Here's how the part is built. I have some questions about the finished solid (model axes, mm). A direction names the side the tool comes from. Round coordinates to 2 decimals unless told otherwise and drop trailing zeros. Write each loop counter-clockwise with the first axis right and the second up, starting at its lowest first coordinate (ties: lowest second). Pieces come first, ordered by that corner, then holes. Notation, with made-up numbers: (23, -0.75) -> (65, -0.75) arc R22 cw to (65, 29.25) -> close; hole circle Ø10 at (55, -7.75). An arc over 180 degrees is marked (long way). Answer in a Markdown table with one row per item. Add a question column.
from build123d import *

# Parameters (mm, degrees)
F4_R     = 3.4
F5_DEPTH = 75.0134427933
F6_SIZE  = 1.5
F7_COUNT = 3


with BuildPart() as f1:
    # F0 (on Front) → F1 (revolve)
    with BuildSketch(Plane.XZ):
        Polygon((-9.15, 1), (-9.15, 25), (-14, 25), (-25, 14.5), (-25, 10.5), (-14, 0), (-10.15, 0), (-10.15, 1), align=None)
    revolve(axis=Axis((0, 0, 12.5), (0, 0, -1)))

    # F2 (on Front) → F3 (revolve)
    with BuildSketch(Plane.XZ):
        Polygon((-35.584796918, -20.8697111031), (-14.8705245175, 0.8309552212), (-10.4189875067, 5.4944701849), (-15.0484629892, 9.9135149637), (-19.5, 5.25), (-40.2142724005, -16.4506663243), align=None)
    revolve(axis=Axis((-29.8571362002, 0, -5.6003331622), (0.6904757467, 0, 0.7233555441)))

    # F4 (on face) → F5 (cut, through all)
    with BuildSketch(Plane(origin=(-27.3888669951, 0, -28.6930987567), x_dir=(0.7233555441, 0, -0.6904757467), z_dir=(-0.6904757467, 0, -0.7233555441))):
        with Locations((-17.7304307809, 0)):
            Circle(F4_R)
    extrude(amount=-F5_DEPTH, mode=Mode.SUBTRACT)

    # F6
    f6_edges = [f1.edges().sort_by_distance(p)[0] for p in [
        (-44.843748, 0, -12.031622),
    ]]
    chamfer(f6_edges, length=F6_SIZE)

    # F7: F1 ×3 about axis
    f7_axis = Axis((0, 0, 14.5), (0, 0, -1))


with BuildPart() as f1_1:
    add(f1.part)
    for i in range(1, F7_COUNT):
        add(f1.part.rotate(f7_axis, i * 360 / F7_COUNT))


solid = f1_1.part
Item 1: If we mould it in two halves opening along X, with no side actions, what happens to faces 3 (the conical face through (-14.01, 4.412, 24.343)), 4 (the cylindrical face through (12.7, -24.61, -7.85)), 5 (the flat face through (9.399, 4.213, 0))? For each: pulls with the +X half, pulls with the -X half, needs draft (parallel to the pull), parting line crosses it, or undercut.
Item 2: If we section it at C-C on z = 18: Please give me the cut outline in (x, y), then the cut area to 3 significant figures.
Item 3: I need wall thicknesses on line 1 along Y through (x, z) = (-35.5, -11.5); line 2 along Y through (x, z) = (0, 14); line 3 along Y through (x, z) = (19, -14). Which ranges of each line are inside material? Lowest first, please. Write a range as from..to.
Item 4: For P1, Ø8, axis at y = -5.5, z = -1, coming from the -X side; P2, Ø3, axis at x = -32.5, z = 2, coming from the +Y side; P3, Ø3, axis at y = 9, z = 13.5, coming from the +X side, each with a flat end and sliding along its axis, tell me the tip position at first contact or that it passes through.
Item 5: On a 3-axis mill with a long thin cutter (end or side, diameter ignored), from which of +Z, -Z, +X, -X, +Y, -Y can I reach the whole of each face in a straight line? I mean faces 1 (the flat face through (3, -9, 25)), 2 (the conical face through (9.691, 16.882, 5.217)). Say none if no direction works.
Item 6: If we section it at A-A on x = 0: Please give me the cut outline in (y, z).
Item 7: If we section it at D-D on z = -8.5: Give the number of separate pieces and of enclosed holes in the cut face, then the cut area to 3 significant figures.
Item 8: If we section it at B-B on y = 0: Please give me the cut outline in (x, z).
Results list:
| question | item | result |
|---|---|---|
| 1 | face 3 | parting line crosses it |
| 1 | face 4 | undercut |
| 1 | face 5 | needs draft |
| 2 | outline | circle Ø42.67 at (0, 0); hole circle Ø18.3 at (0, 0) |
| 2 | area | 1,170 mm² |
| 3 | line 1 | -6.4..-3.4, 3.4..6.4 |
| 3 | line 2 | -25..-9.15, 9.15..25 |
| 3 | line 3 | -38.43..-37.06, -28.58..-24.84, 24.84..28.58, 37.06..38.43 |
| 4 | P1 | x = -36.26 |
| 4 | P2 | y = 2.99 |
| 4 | P3 | x = 23.85 |
| 5 | face 1 | +Z, +X, -X, +Y, -Y |
| 5 | face 2 | none |
| 6 | outline | (-25, 10.5) -> (-14, 0) -> (-10.15, 0) -> (-10.15, 1) -> (-9.15, 1) -> (-9.15, 25) -> (-14, 25) -> (-25, 14.5) -> close; (9.15, 1) -> (10.15, 1) -> (10.15, 0) -> (14, 0) -> (25, 10.5) -> (25, 14.5) -> (14, 25) -> (9.15, 25) -> close |
| 7 | separate pieces | 3 |
| 7 | enclosed holes | 3 |
| 7 | area | 383 mm² |
| 8 | outline | (-43.81, -10.95) -> (-43.76, -13.07) -> (-42.67, -14.1) -> (-21.96, 7.6) -> (-17.04, 2.9) -> (-37.75, -18.8) -> (-36.67, -19.83) -> (-34.55, -19.78) -> (-14.87, 0.83) -> (-14, 0) -> (-10.15, 0) -> (-10.15, 1) -> (-9.15, 1) -> (-9.15, 25) -> (-14, 25) -> (-25, 14.5) -> (-25, 10.5) -> (-24.13, 9.67) -> close; (9.15, 1) -> (10.15, 1) -> (10.15, 0) -> (14, 0) -> (25, 10.5) -> (25, 14.5) -> (14, 25) -> (9.15, 25) -> close |
